Drawing for the job (mm, zero at the part's lowest x, y, z). A direction names the side the tool comes from. Round coordinates to 2 decimals unless told otherwise and drop trailing zeros. Write each loop counter-clockwise with the first axis right and the second up, starting at its lowest first coordinate (ties: lowest second). Pieces come first, ordered by that corner, then holes. Notation, with made-up numbers: (33.25, 3) -> (53.25, 3) arc R31 cw to (53.25, 29) -> close; hole circle Ø7 at (36.25, -31.75). An arc over 180 degrees is marked (long way). One line per question, with ' | ' between items.
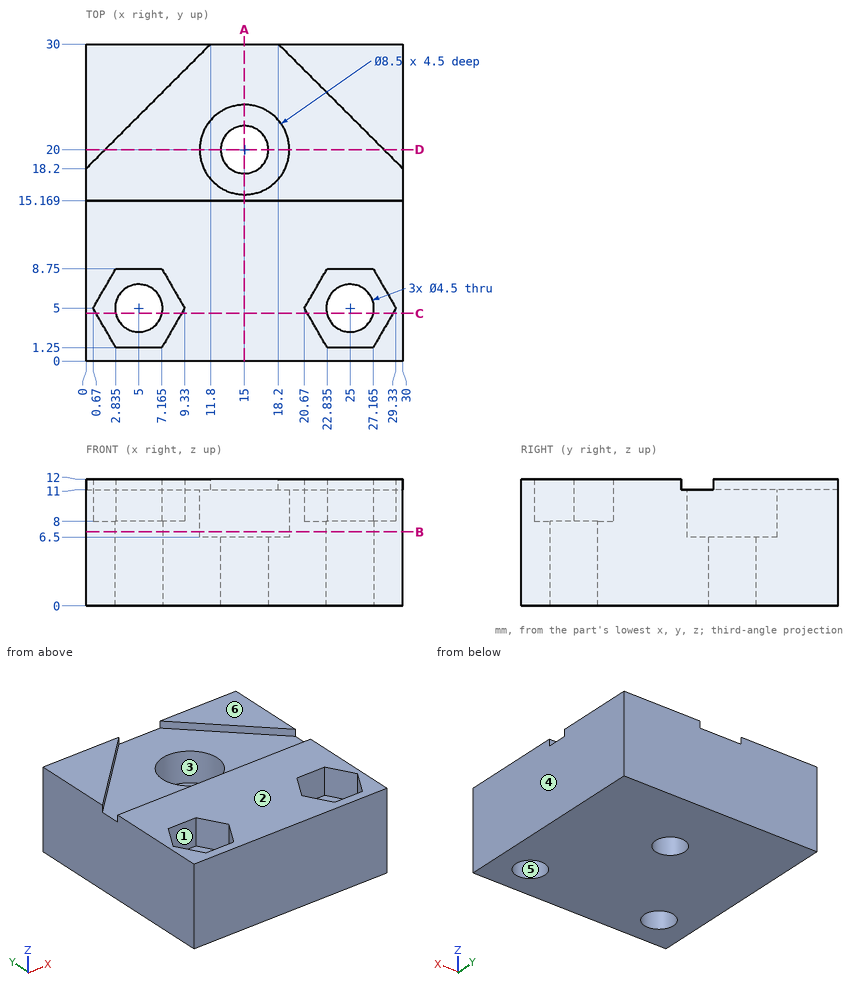
(1) Mould opens along X. For the marked faces 3, 4, 5 and 6 say: pulls with the +X half, pulls with the -X half, needs draft (parallel to the pull), parting line crosses it, or undercut.
Calculated:
face 3: undercut | face 4: pulls with the +X half | face 5: undercut | face 6: needs draft
(2) 3-axis set-ups, long thin cutter, end or side, ignore diameter. For the marked faces 1 and 2: which of +Z, -Z, +X, -X, +Y, -Y reach the whole face in a straight line?
Calculated:
face 1: +Z | face 2: +Z, +X, -X, +Y, -Y
(3) Slice it at B-B (z = 7). Write the cut outline in (x, y).
Calculated:
outline: (0, 0) -> (30, 0) -> (30, 30) -> (0, 30) -> close; hole circle Ø4.5 at (5, 5); hole circle Ø8.5 at (15, 20); hole circle Ø4.5 at (25, 5)
(4) Slice it at C-C (y = 4.5). Write the cut outline in (x, z), then the cut area to 3 significant figures.
Calculated:
outline: (0, 0) -> (2.81, 0) -> (2.81, 8) -> (0.96, 8) -> (0.96, 12) -> (0, 12) -> close; (7.19, 0) -> (22.81, 0) -> (22.81, 8) -> (20.96, 8) -> (20.96, 12) -> (9.04, 12) -> (9.04, 8) -> (7.19, 8) -> close; (27.19, 0) -> (30, 0) -> (30, 12) -> (29.04, 12) -> (29.04, 8) -> (27.19, 8) -> close | area: 225 mm2
(5) Wall check: line 1 (Y direction, x = 3, z = 8.5); line 2 (Y direction, x = 15, z = 5); line 3 (X direction, y = 4.5, z = 6.5). Give the ranges that are in metal, low to high. Write a range as from..to.
Calculated:
line 1: 0..1.25, 8.75..30 | line 2: 0..17.75, 22.25..30 | line 3: 0..2.81, 7.19..22.81, 27.19..30
(6) Slice it at D-D (y = 20). Write the cut outline in (x, z).
Calculated:
outline: (0, 0) -> (12.75, 0) -> (12.75, 6.5) -> (10.75, 6.5) -> (10.75, 11) -> (1.8, 11) -> (1.8, 12) -> (0, 12) -> close; (17.25, 0) -> (30, 0) -> (30, 12) -> (28.2, 12) -> (28.2, 11) -> (19.25, 11) -> (19.25, 6.5) -> (17.25, 6.5) -> close
(7) Slice it at A-A (x = 15). Write the cut outline in (y, z).
Calculated:
outline: (0, 0) -> (17.75, 0) -> (17.75, 6.5) -> (15.75, 6.5) -> (15.75, 11) -> (15.17, 11) -> (15.17, 12) -> (0, 12) -> close; (22.25, 0) -> (30, 0) -> (30, 11) -> (24.25, 11) -> (24.25, 6.5) -> (22.25, 6.5) -> close
(8) Drop flat-ended pins along their axis: pin 1 (6 mm diameter, centred on x = 3.5, y = 6.5, fed in from -Z); pin 2 (5 mm diameter, centred on x = 25, y = 5, fed in from +Z); pin 3 (2.5 mm diameter, centred on x = 13.5, y = 20.5, fed in from +Z). Give the stop position or say it passes through.
Calculated:
pin 1: z = 0 | pin 2: z = 8 | pin 3: z = 6.5
